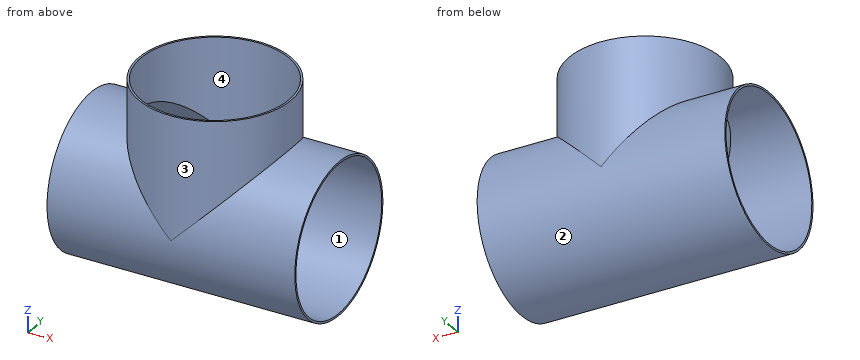
Autodesk Inventor part; units mm, degrees
ref_plane "YZ Plane" through (0, 0, 0) normal (1, 0, 0) x (0, 1, 0)
ref_plane "XZ Plane" through (0, 0, 0) normal (0, 1, 0) x (-1, 0, 0)
ref_plane "XY Plane" through (0, 0, 0) normal (0, 0, 1) x (1, 0, 0)
sketch "Sketch1" plane through (0, 0, 0) normal (1, 0, 0) x (0, 1, 0)
  circle A0 centre (0, 0) radius 109.55
  dimension "d0" = 219.1
extrude "Extrude1" add sketch "Sketch1" along normal blind 356
sketch "Sketch2" plane through (0, 0, 0) normal (0, 0, 1) x (1, 0, 0)
  line L0 (0, 109.55) -> (0, -109.55)
  line L1 (356, 109.55) -> (356, -109.55)
  line L2 (0, 0) -> (356, 0) construction
  circle A0 centre (178, 0) radius 109.55
  dimension "d3" = 219.1
extrude "Extrude2" add sketch "Sketch2" along normal blind 178
sketch "Sketch3" plane through (0, 0, 0) normal (-1, 0, 0) x (0, 0, 1)
  circle A0 centre (0, 0) radius 109.55
  circle A1 centre (0, 0) radius 106.65
  dimension "d6" = 213.3
extrude "Extrude3" cut sketch "Sketch3" against normal through all contours A1
sketch "Sketch4" plane through (178, 0, 178) normal (0, 0, 1) x (1, 0, 0)
  circle A0 centre (0, 0) radius 109.55
  circle A1 centre (0, 0) radius 106.65
  dimension "d9" = 213.3
extrude "Extrude4" cut sketch "Sketch4" against normal up to next contours A1
equation "\"d0\" = d"
equation "\"d1\" = 2 * a"
equation "\"d3\" = d"
equation "\"d4\" = a"
equation "\"d6\" = d - 2 * s1"
equation "\"d7\" = a"
equation "\"d9\" = d - 2 * s1"
equation "\"d10\" = a"
equation "\"d\" = 219.1"
equation "\"s1\" = 2.9"
equation "\"a\" = 178"
equation "\"Size_Designation\" = 1.2345"
properties part number "DIN 2615-1 Tee 219.1 x 2.9 S" material "Steel"
Read the model definition and answer for the solid it produces. Units are mm, in the model's axes. Face numbers are marked on the shaded views. A direction names the side the tool comes from. Coordinates: 2 decimals unless noted, no trailing zeros. Write each loop counter-clockwise with the first axis right and the second up, starting at its lowest first coordinate (ties: lowest second). Pieces come first, ordered by that corner, then holes. Notation, with made-up numbers: (9, 73) -> (23, 73) arc R18 cw to (23, 92) -> close; hole circle Ø11 at (44.5, 5). An arc over 180 degrees is marked (long way). Answer as a JSON object with one key per item and string values.
Q1. Flat-ended cylindrical pins translate along their axes: pin 1 Ø4 at (x, y) = (165.5, -18) entering from -Z; pin 2 Ø5 at (x, y) = (143, 65.5) entering from +Z; pin 3 Ø5 at (x, y) = (245.5, 21) entering from -Z. Find the tip coordinate at first contact, or state that the pin passes through.
The answers:
{"pin 1": "stops at z = -108.38", "pin 2": "stops at z = -82.16", "pin 3": "stops at z = -107.98"}
Q2. Determine the mould class of the marked faces 3 and 4 for opening direction X: pulls with the +X half, pulls with the -X half, needs draft (parallel to the pull), parting line crosses it, or undercut.
The answers:
{"face 3": "parting line crosses it", "face 4": "undercut"}
Q3. The part is cut by section B-B on z = -79.5. Give the vertices of the cut face in (x, y).
The answers:
{"outline": "(0, -75.37) -> (356, -75.37) -> (356, -71.09) -> (0, -71.09) -> close; (0, 71.09) -> (356, 71.09) -> (356, 75.37) -> (0, 75.37) -> close"}
Q4. The part is cut by section C-C on x = 178. Give the vertices of the cut face in (y, z).
The answers:
{"outline": "(-109.55, 0) arc R109.55 ccw to (109.55, 0) -> (109.55, 178) -> (106.65, 178) -> (106.65, 0) arc R106.65 cw to (-106.65, 0) -> (-106.65, 178) -> (-109.55, 178) -> close"}
Q5. Consider line 1 (Y direction, x = 178, z = 115); line 2 (X direction, y = 0, z = 136); line 3 (X direction, y = 26, z = 145.5). Determine where each line is inside the solid, lowest interval first. Write a range as [from, to].
The answers:
{"line 1": "y = [-109.55, -106.65], [106.65, 109.55]", "line 2": "x = [68.45, 71.35], [284.65, 287.55]", "line 3": "x = [71.58, 74.57], [281.43, 284.42]"}
Q6. The part is cut by section D-D on z = 17. Give the vertices of the cut face in (x, y).
The answers:
{"outline": "(0, -108.22) -> (161, -108.22) arc R109.55 ccw to (195, -108.22) -> (356, -108.22) -> (356, -105.29) -> (195, -105.29) arc R106.65 cw to (161, -105.29) -> (0, -105.29) -> close; (0, 105.29) -> (161, 105.29) arc R106.65 cw to (195, 105.29) -> (356, 105.29) -> (356, 108.22) -> (195, 108.22) arc R109.55 ccw to (161, 108.22) -> (0, 108.22) -> close"}
Q7. A tool of negligible diameter and unlimited length cuts with its end or side. For the marked faces 1 and 2, from which of +Z, -Z, +X, -X, +Y, -Y can it reach the whole face along a straight path? Write none if from no direction.
The answers:
{"face 1": "+X, -X", "face 2": "none"}
Q8. The part is cut by section A-A on y = 0. Give the vertices of the cut face in (x, z), then the cut area to 3 significant figures.
The answers:
{"outline": "(0, -109.55) -> (356, -109.55) -> (356, -106.65) -> (0, -106.65) -> close; (0, 106.65) -> (71.35, 106.65) -> (71.35, 178) -> (68.45, 178) -> (68.45, 109.55) -> (0, 109.55) -> close; (284.65, 106.65) -> (356, 106.65) -> (356, 109.55) -> (287.55, 109.55) -> (287.55, 178) -> (284.65, 178) -> close", "area": "1,840 mm2"}
